The model under review builds one solid part; all positions refer to its coordinate system, in mm. Face numbers are marked on the shaded views. A direction names the side the tool comes from. Round coordinates to 2 decimals unless told otherwise and drop trailing zeros. Write each loop counter-clockwise with the first axis right and the second up, starting at its lowest first coordinate (ties: lowest second). Pieces come first, ordered by that corner, then holes. Notation, with made-up numbers: (-31, 72.5) - (6, 72.5) arc R14 cw to (6, 84.5) - close; hole circle Ø11 at (12.25, 9). An arc over 180 degrees is marked (long way). Write each question's results on one line, items separated by ' | '.
```python
from build123d import *

# Parameters (mm, degrees)
JOTYY_MIRRORED_START         = -10
JOTYY_MIRRORED_OUTLINE_W     = 53.8
JOTYY_MIRRORED_OUTLINE_H     = 36
JOTYY_MIRRORED_OUTLINE_R     = 2.1
JOTYY_MIRRORED_OUTLINE_R_2   = 11
JOTYY_MIRRORED_DEPTH         = 10
JOTYY_MIRRORED_2_OUTLINE_R   = 11
JOTYY_MIRRORED_2_OUTLINE_R_2 = 4
JOTYY_MIRRORED_2_DEPTH       = 2.5
SKETCH1_R                    = 4
CUT_EXTRUDE1_DEPTH           = 10


# Read off the part's stored shape, not the designer's step: jotyy_Mirrored
with BuildPart() as part:
    # jotyy_Mirrored outline → jotyy_Mirrored (new body)
    with BuildSketch(Plane.XY.offset(JOTYY_MIRRORED_START)):
        with Locations((-26.9, 20)):
            Rectangle(JOTYY_MIRRORED_OUTLINE_W, JOTYY_MIRRORED_OUTLINE_H)
        with Locations((-47.5, 7.5)):
            Circle(JOTYY_MIRRORED_OUTLINE_R, mode=Mode.SUBTRACT)
        with Locations((-22.5, 7.5)):
            Circle(JOTYY_MIRRORED_OUTLINE_R, mode=Mode.SUBTRACT)
        with Locations((-5, 7.5)):
            Circle(JOTYY_MIRRORED_OUTLINE_R, mode=Mode.SUBTRACT)
        with Locations((-35, 20)):
            Circle(JOTYY_MIRRORED_OUTLINE_R_2, mode=Mode.SUBTRACT)
        with Locations((-47.5, 32.5)):
            Circle(JOTYY_MIRRORED_OUTLINE_R, mode=Mode.SUBTRACT)
        with Locations((-22.5, 32.5)):
            Circle(JOTYY_MIRRORED_OUTLINE_R, mode=Mode.SUBTRACT)
        with Locations((-5, 32.5)):
            Circle(JOTYY_MIRRORED_OUTLINE_R, mode=Mode.SUBTRACT)
    extrude(amount=JOTYY_MIRRORED_DEPTH)

    # jotyy_Mirrored 2 outline → jotyy_Mirrored 2 (add)
    with BuildSketch(Plane.XY.offset(JOTYY_MIRRORED_START)):
        with Locations((-35, 20)):
            Circle(JOTYY_MIRRORED_2_OUTLINE_R)
        with Locations((-35, 20)):
            Circle(JOTYY_MIRRORED_2_OUTLINE_R_2, mode=Mode.SUBTRACT)
    extrude(amount=JOTYY_MIRRORED_2_DEPTH)

    # Sketch1 → Cut-Extrude1 (cut)
    with BuildSketch(Plane.XY):
        with Locations((-10, 20)):
            Circle(SKETCH1_R)
    extrude(amount=-CUT_EXTRUDE1_DEPTH, mode=Mode.SUBTRACT)


solid = part.part
```
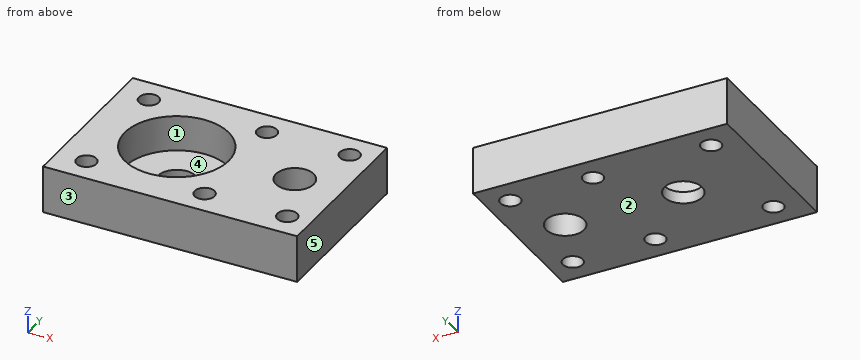
Q1. We need section B-B (y = 20). State the section outline as (x, z) points.
Evaluation:
outline: (-53.8, -10) - (-39, -10) - (-39, -7.5) - (-46, -7.5) - (-46, 0) - (-53.8, 0) - close; (-31, -10) - (-14, -10) - (-14, 0) - (-24, 0) - (-24, -7.5) - (-31, -7.5) - close; (-6, -10) - (0, -10) - (0, 0) - (-6, 0) - close
Q2. For probe 1 along Y at (x, z) = (-47.5, -4); probe 2 along X at (y, z) = (20.5, -1.5); probe 3 along Y at (x, z) = (-35, -8.2), list the stretches that pass through material, from the lowest coordinate up.
Evaluation:
probe 1: y = 2 to 5.4, 9.6 to 30.4, 34.6 to 38 | probe 2: x = -53.8 to -45.99, -24.01 to -13.97, -6.03 to 0 | probe 3: y = 2 to 16, 24 to 38
Q3. The part is to be moulded in two halves that separate along Y. For the marked faces 3, 4 and 5, say which applies: released by +Y, released by -Y, zero draft, split by the parting line, or undercut.
Evaluation:
face 3: released by -Y | face 4: undercut | face 5: zero draft
Q4. We need section C-C (x = -22.5). State the section outline as (y, z) points, plus the area to 3 significant figures.
Evaluation:
outline: (2, -10) - (5.4, -10) - (5.4, 0) - (2, 0) - close; (9.6, -10) - (30.4, -10) - (30.4, 0) - (9.6, 0) - close; (34.6, -10) - (38, -10) - (38, 0) - (34.6, 0) - close | area: 276 mm^2
Q5. Tool access review of the marked faces 1 and 2: name each direction out of +Z, -Z, +X, -X, +Y, -Y from which nothing blocks a thin tool from reaching the whole face with its end or side.
Evaluation:
face 1: +Z | face 2: -Z, +X, -X, +Y, -Y
Q6. We need section A-A (x = -10). State the section outline as (y, z) points, plus the area to 3 significant figures.
Evaluation:
outline: (2, -10) - (16, -10) - (16, 0) - (2, 0) - close; (24, -10) - (38, -10) - (38, 0) - (24, 0) - close | area: 280 mm^2
Q7. Insertion check: P1, Ø4, axis at x = -47.5, y = 32.5, coming from the +Z side. The pin has a flat end and moves straight along its axis. Give the tip position at first contact, or say it passes through.
Evaluation:
P1: passes through
Q8. We need section D-D (y = 7.5). State the section outline as (x, z) points, plus the area to 3 significant figures.
Evaluation:
outline: (-53.8, -10) - (-49.6, -10) - (-49.6, 0) - (-53.8, 0) - close; (-45.4, -10) - (-24.6, -10) - (-24.6, 0) - (-45.4, 0) - close; (-20.4, -10) - (-7.1, -10) - (-7.1, 0) - (-20.4, 0) - close; (-2.9, -10) - (0, -10) - (0, 0) - (-2.9, 0) - close | area: 412 mm^2
